Answer from the drawing. Dimensions are ordinates in mm from the lowest x, y and z of the part. Round coordinates to 2 decimals unless told otherwise and drop trailing zeros. Write each loop counter-clockwise with the first axis right and the second up, starting at its lowest first coordinate (ties: lowest second). Pieces come first, ordered by that corner, then holes. Notation, with made-up numbers: (85.25, 55) -> (89.25, 55) arc R31 ccw to (89.25, 80) -> close; hole circle Ø2 at (-8, 17). An arc over 180 degrees is marked (long way). Return JSON: item names as keys, results as strings. Group by question number.
(1) Given pin 1 (3 mm diameter, centred on x = 5, z = 71.7, fed in from -Y); pin 2 (0.9 mm diameter, centred on x = 114, y = 1, fed in from -Z); pin 3 (1.5 mm diameter, centred on x = 57.5, y = 1, fed in from -Z); pin 4 (0.9 mm diameter, centred on y = 2, z = 38.5, fed in from +X), each flat-ended and moving along its own axis, determine where each tip first touches the part or whether it passes through.
(2) A cutting plane is placed at D-D on x = 114. Give the vertices of the cut face in (y, z), then the cut area to 3 significant figures.
(3) A cutting plane is placed at A-A on y = 1.4. Give the vertices of the cut face in (x, z), then the cut area to 3 significant figures.
(4) A cutting plane is placed at C-C on z = 41. Give the vertices of the cut face in (x, y).
(5) A cutting plane is placed at B-B on z = 21. Give the vertices of the cut face in (x, y).
(6) Straight lines are drawn through the part: line 1 (Z direction, x = 58.5, y = 2.7); line 2 (Z direction, x = 108, y = 1.8); line 3 (Z direction, x = 89, y = 0.9). For each, find the intervals that lie inside material, in ascending order.
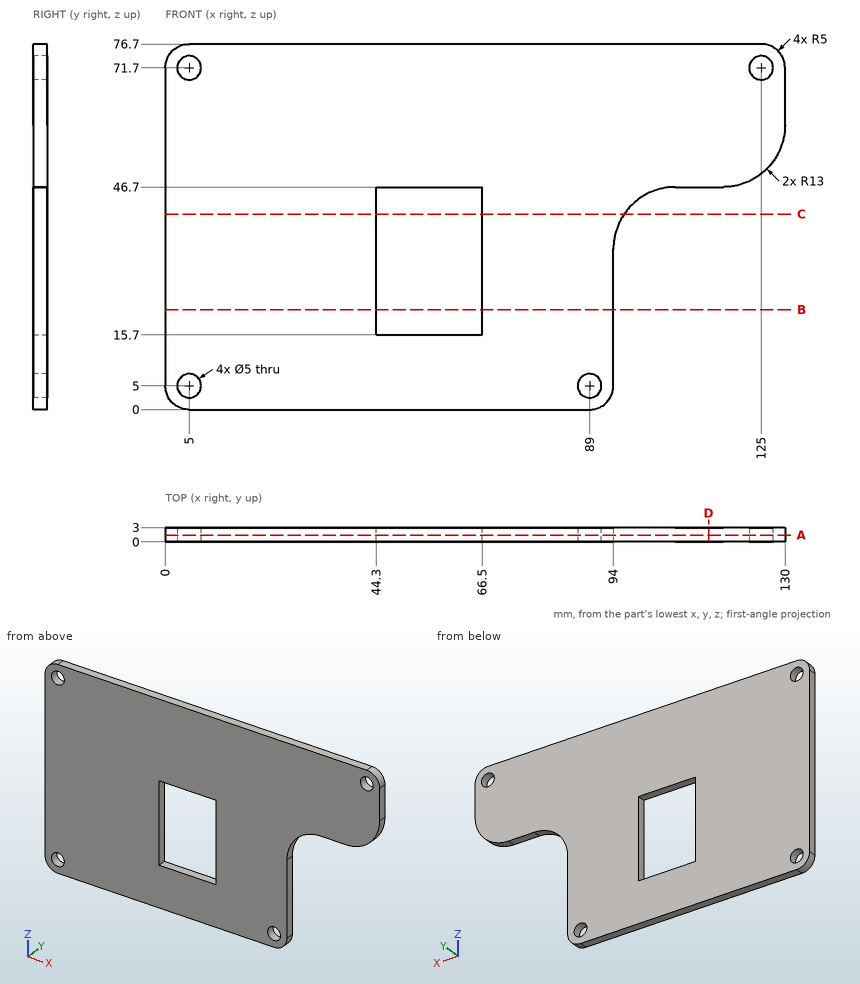
Checks:
{
 "1": {"pin 1": "passes through", "pin 2": "stops at z = 46.7", "pin 3": "stops at z = 0", "pin 4": "stops at x = 95.11"},
 "2": {"outline": "(0, 46.7) -> (3, 46.7) -> (3, 76.7) -> (0, 76.7) -> close", "area": "90.0 mm^2"},
 "3": {"outline": "(0, 5) arc R5 ccw to (5, 0) -> (89, 0) arc R5 ccw to (94, 5) -> (94, 33.7) arc R13 cw to (107, 46.7) -> (117, 46.7) arc R13 ccw to (130, 59.7) -> (130, 71.7) arc R5 ccw to (125, 76.7) -> (5, 76.7) arc R5 ccw to (0, 71.7) -> close; hole circle Ø5 at (5, 5); hole circle Ø5 at (5, 71.7); hole (44.3, 15.7) -> (66.5, 15.7) -> (66.5, 46.7) -> (44.3, 46.7) -> close; hole circle Ø5 at (89, 5); hole circle Ø5 at (125, 71.7)", "area": "7,500 mm^2"},
 "4": {"outline": "(0, 0) -> (44.3, 0) -> (44.3, 3) -> (0, 3) -> close; (66.5, 0) -> (96.24, 0) -> (96.24, 3) -> (66.5, 3) -> close"},
 "5": {"outline": "(0, 0) -> (44.3, 0) -> (44.3, 3) -> (0, 3) -> close; (66.5, 0) -> (94, 0) -> (94, 3) -> (66.5, 3) -> close"},
 "6": {"line 1": "z = 0 to 15.7, 46.7 to 76.7", "line 2": "z = 46.7 to 76.7", "line 3": "z = 0 to 2.5, 7.5 to 76.7"}
}
